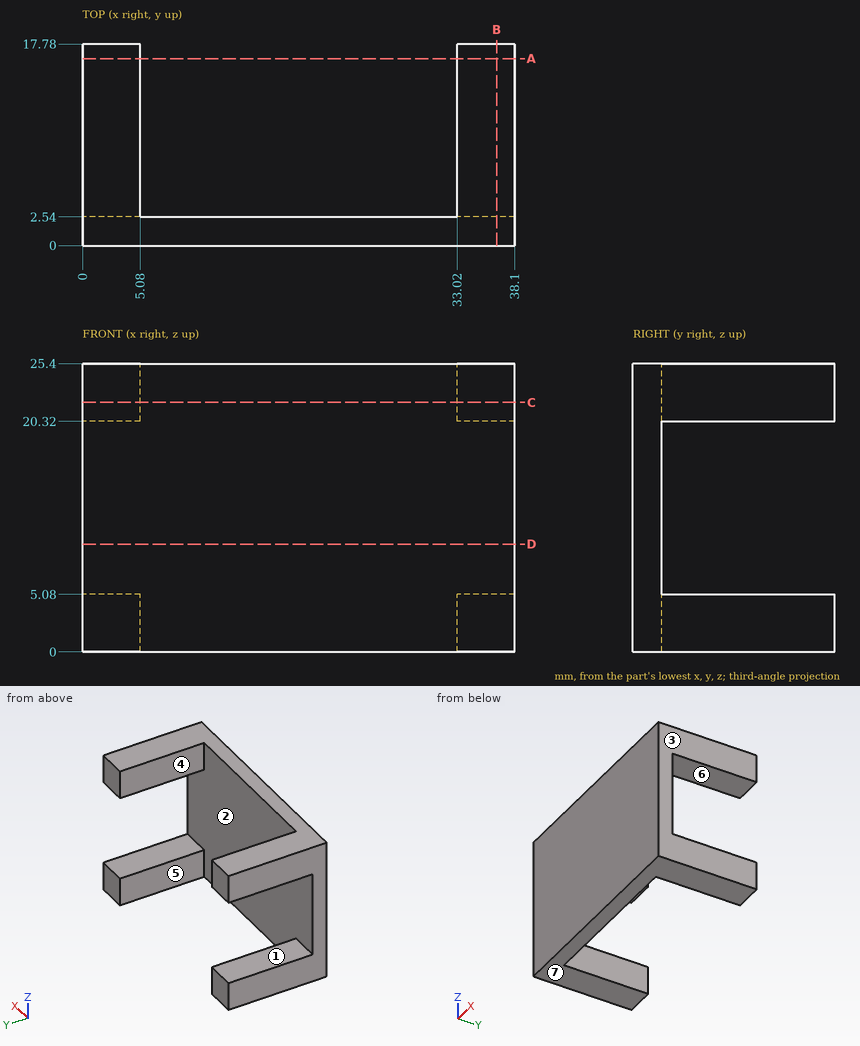
Here's the drawing with two shaded views (mm, measured from the low corner). I have some questions. A direction names the side the tool comes from. Give positions to 0.01 mm unless a question says otherwise; leave off trailing zeros. Order: outer loops, then holes, each group sorted by start corner. A loop starts at its lowest first (then second) coordinate and runs counter-clockwise, first axis right, second up. Notation, with made-up numbers: (64, 59.5) - (101, 59.5) arc R31 cw to (101, 89.5) - close; hole circle Ø4 at (25, 52.25). An arc over 180 degrees is marked (long way). Use a Markdown table: item, result. Add a question column.
Q1. If we section it at B-B on x = 36.5: Write out the boundary of the cut face in (y, z), plus the area to 3 significant figures.
Q2. If we section it at C-C on z = 22: Write out the boundary of the cut face in (x, y).
Q3. If we mould it in two halves opening along X, with no side actions, what happens to the marked faces 1, 2, 3 and 4? For each: released by +X, released by -X, zero draft, split by the parting line, or undercut.
Q4. Please list where these lines run through material, in increasing order: line 1 along Z through (x, y) = (4, 2.75); line 2 along Y through (x, z) = (27.5, 23.75).
Q5. I'm going to push a flat-ended pin straight in: pin 1 (7.5 mm diameter, centred on x = 10.5, z = 7, fed in from +Y). Where does the tip first touch, or does it pass through?
Q6. On a 3-axis mill with a long thin cutter (end or side, diameter ignored), from which of +Z, -Z, +X, -X, +Y, -Y can I reach the whole of each face in a straight line? I mean the marked faces 5, 6 and 7. Say none if no direction works.
Q7. If we section it at D-D on z = 9.5: Write out the boundary of the cut face in (x, y), plus the area to 3 significant figures.
Q8. If we section it at A-A on y = 16.5: Write out the boundary of the cut face in (x, z).
Answers follow:
| question | item | result |
|---|---|---|
| 1 | outline | (0, 0) - (17.78, 0) - (17.78, 5.08) - (2.54, 5.08) - (2.54, 20.32) - (17.78, 20.32) - (17.78, 25.4) - (0, 25.4) - close |
| 1 | area | 219 mm^2 |
| 2 | outline | (0, 0) - (38.1, 0) - (38.1, 17.78) - (33.02, 17.78) - (33.02, 2.54) - (5.08, 2.54) - (5.08, 17.78) - (0, 17.78) - close |
| 3 | face 1 | zero draft |
| 3 | face 2 | undercut |
| 3 | face 3 | released by +X |
| 3 | face 4 | undercut |
| 4 | line 1 | z = 0 to 5.08, 20.32 to 25.4 |
| 4 | line 2 | y = 0 to 2.54 |
| 5 | pin 1 | stops at y = 2.54 |
| 6 | face 5 | +Z, -Z, +Y |
| 6 | face 6 | +X, -X, +Y |
| 6 | face 7 | -Z, +X, -X, +Y, -Y |
| 7 | outline | (0, 0) - (38.1, 0) - (38.1, 2.54) - (0, 2.54) - close |
| 7 | area | 96.8 mm^2 |
| 8 | outline | (0, 0) - (5.08, 0) - (5.08, 5.08) - (0, 5.08) - close; (0, 20.32) - (5.08, 20.32) - (5.08, 25.4) - (0, 25.4) - close; (33.02, 0) - (38.1, 0) - (38.1, 5.08) - (33.02, 5.08) - close; (33.02, 20.32) - (38.1, 20.32) - (38.1, 25.4) - (33.02, 25.4) - close |
